Here's how the part is built. I have some questions about the finished solid (model axes, mm). Round coordinates to 2 decimals unless told otherwise and drop trailing zeros. Write each loop counter-clockwise with the first axis right and the second up, starting at its lowest first coordinate (ties: lowest second). Pieces come first, ordered by that corner, then holes. Notation, with made-up numbers: (-26.75, 58) - (-5.75, 58) arc R23 cw to (-5.75, 80) - close; hole circle Ø5 at (42, -32.5). An arc over 180 degrees is marked (long way). Write item = value, one per line. Start each with the question number.
Item 1: If we section it at A-A (y = -15.25): Please give me the cut outline in (x, z), and give its area (3 significant figures).
Item 2: If we section it at B-B (x = -0.25): Please give me the cut outline in (y, z), and give its area (4 significant figures).
Item 3: If I drill on line 1 along Y through (x, z) = (-1, -2.5), over which ranges is the centre line in solid material (lowest first)? Write a range as [from, to].
Item 4: If we section it at C-C (z = -2.5): Please give me the cut outline in (x, y).
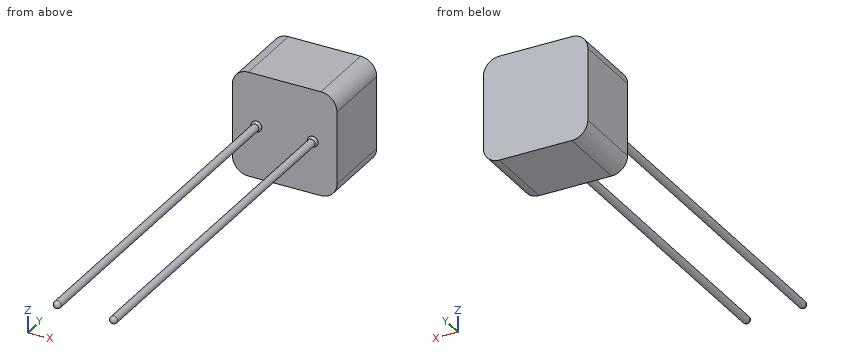
Autodesk Inventor part; units mm, degrees
ref_plane "YZ Plane" through (0, 0, 0) normal (1, 0, 0) x (0, 1, 0)
ref_plane "XZ Plane" through (0, 0, 0) normal (0, 1, 0) x (-1, 0, 0)
ref_plane "XY Plane" through (0, 0, 0) normal (0, 0, 1) x (1, 0, 0)
sketch "Sketch1" plane through (0, 0, 0) normal (0, 1, 0) x (-1, 0, 0)
  line L0 (2.25, 3.25) -> (-2.25, 3.25)
  line L1 (-3.25, 2.25) -> (-3.25, -2.25)
  line L2 (-2.25, -3.25) -> (2.25, -3.25)
  line L3 (3.25, -2.25) -> (3.25, 2.25)
  line L4 (3.25, 3.25) -> (-3.25, -3.25) construction
  line L5 (-3.25, 3.25) -> (3.25, -3.25) construction
  arc A0 (-3.25, -2.25) -> (-2.25, -3.25) centre (-2.25, -2.25) ccw
  arc A1 (2.25, -3.25) -> (3.25, -2.25) centre (2.25, -2.25) ccw
  arc A2 (3.25, 2.25) -> (2.25, 3.25) centre (2.25, 2.25) ccw
  arc A3 (-2.25, 3.25) -> (-3.25, 2.25) centre (-2.25, 2.25) ccw
  point P0 (0, 0)
  dimension "d0" = 6.5
  dimension "d1" = 6.5
  dimension "d4" = 1
extrude "Extrusion1" add sketch "Sketch1" along normal mid plane 4.5
sketch "Sketch4" plane through (0, 0, 0) normal (0, 0, 1) x (1, 0, 0)
  arc A0 (-1.75, -25) -> (-1.5182, -24.7516) centre (-1.7559, -24.7621) ccw
  line L0 (-1.75, -2.4144) -> (-1.75, -25)
  line L1 (-1.5182, -2.4144) -> (-1.5182, -24.7516)
  arc A1 (-1.5182, -2.4144) -> (-1.4227, -2.25) centre (-1.6226, -2.2437) ccw
  line L2 (-1.75, -2.4144) -> (-1.75, -2.25)
  line L3 (-1.75, -2.25) -> (-1.4227, -2.25)
  point P0 (0, 0)
  dimension "d27" = 0.2
revolve "Revolution2" add sketch "Sketch4" angle 360 about axis through (-1.75, -2.4144, 0) along (0, -1, 0)
pattern_linear "Rectangular Pattern4" count 2 spacing 3.5 along (1, 0, 0) of "Revolution2"
properties part number "A54"
Reply:
q1.outline = circle Ø0.46 at (-1.75, 0); circle Ø0.46 at (1.75, 0)
q1.area = 0.338 mm2
q2.outline = (-2.25, -3.25) - (2.25, -3.25) - (2.25, 3.25) - (-2.25, 3.25) - close
q2.area = 29.25 mm2
q3.line_1 = [-2.25, 2.25]
q4.outline = (-3.22, -2.25) - (3.22, -2.25) - (3.22, 2.25) - (-3.22, 2.25) - close
